Could you check a few things on this model? Use its own coordinates, in mm. A direction names the side the tool comes from. Coordinates: 2 decimals unless noted, no trailing zeros. Write each loop counter-clockwise with the first axis right and the second up, starting at its lowest first coordinate (ties: lowest second). Pieces come first, ordered by that corner, then holes. Notation, with made-up numbers: M 40,52 L 97,52 A13 cw 97,71 Z; hole C 74.25,-35.75 d1. An arc over 180 degrees is marked long. Write item = value, one per line.
```python
from build123d import *

# Parameters (mm, degrees)
F1_DEPTH = 12.7
F2_W     = 12.7
F2_H     = 76.2
F3_DEPTH = 50.8


with BuildPart() as f1:
    # F0 (on Front) → F1 (new body)
    with BuildSketch(Plane.XZ):
        Polygon((36.304801, 33.762489), (-27.195199, 33.762489), (-27.195199, 8.362489), (-1.795199, 8.362489), (-1.795199, -4.337511), (-14.495199, -4.337511), (-14.495199, -17.037511), (10.904801, -17.037511), (10.904801, -42.437511), (36.304801, -42.437511), align=None)
    extrude(amount=F1_DEPTH)

    # F2 (on face) → F3 (join)
    with BuildSketch(Plane.XZ.offset(12.7)):
        with Locations((29.954801, -4.337511)):
            Rectangle(F2_W, F2_H)
    extrude(amount=F3_DEPTH)


solid = f1.part
```
Item 1: Imagine slicing it at D-D (x = 9.5). Write out the boundary of the cut face in (y, z), and give its area (3 significant figures).
Numbers:
outline = M -12.7,-17.04 L 0,-17.04 L 0,33.76 L -12.7,33.76 Z
area = 645 mm²
Item 2: If I drill on line 1 along X through (y, z) = (-45, -15.5); line 2 along Y through (x, z) = (-9, -7.5), over which ranges is the centre line in solid material (lowest first)?
Numbers:
line_1 = 23.6 to 36.3
line_2 = -12.7 to 0
Item 3: I'm going to push flat-ended pins straight in: P1, Ø12, axis at x = 22.5, y = -16, coming from the -Z side; P2, Ø10, axis at x = -1.5, y = -3.5, coming from the -Z side; P3, Ø12, axis at y = -51.5, z = -5, coming from the -X side; P4, Ø4, axis at y = -9, z = 3, coming from the -X side. Where does each tip first touch, or does it pass through?
Numbers:
P1 = -42.44
P2 = -17.04
P3 = 23.6
P4 = -1.8
Item 4: Imagine slicing it at B-B (y = -11). Write out the boundary of the cut face in (x, z).
Numbers:
outline = M -27.2,8.36 L -1.8,8.36 L -1.8,-4.34 L -14.5,-4.34 L -14.5,-17.04 L 10.9,-17.04 L 10.9,-42.44 L 36.3,-42.44 L 36.3,33.76 L -27.2,33.76 Z
Item 5: For faces 1 (the face through (-14.495, -6, -11)), 2 (the face through (-15, -6, 8.362)), 3 (the face through (23.605, -38, -5)), which set-ups out of +Z, -Z, +X, -X, +Y, -Y let a thin tool reach every point of the face, with its end or its side?
Numbers:
face_1 = -Z, -X, +Y, -Y
face_2 = -X, +Y, -Y
face_3 = +Z, -Z, -X, -Y
Item 6: Imagine slicing it at C-C (z = 19). Write out the boundary of the cut face in (x, y).
Numbers:
outline = M -27.2,-12.7 L 23.6,-12.7 L 23.6,-63.5 L 36.3,-63.5 L 36.3,0 L -27.2,0 Z
Item 7: Imagine slicing it at A-A (x = -12.5). Write out the boundary of the cut face in (y, z), and give its area (3 significant figures).
Numbers:
outline = M -12.7,-17.04 L 0,-17.04 L 0,-4.34 L -12.7,-4.34 Z; M -12.7,8.36 L 0,8.36 L 0,33.76 L -12.7,33.76 Z
area = 484 mm²
